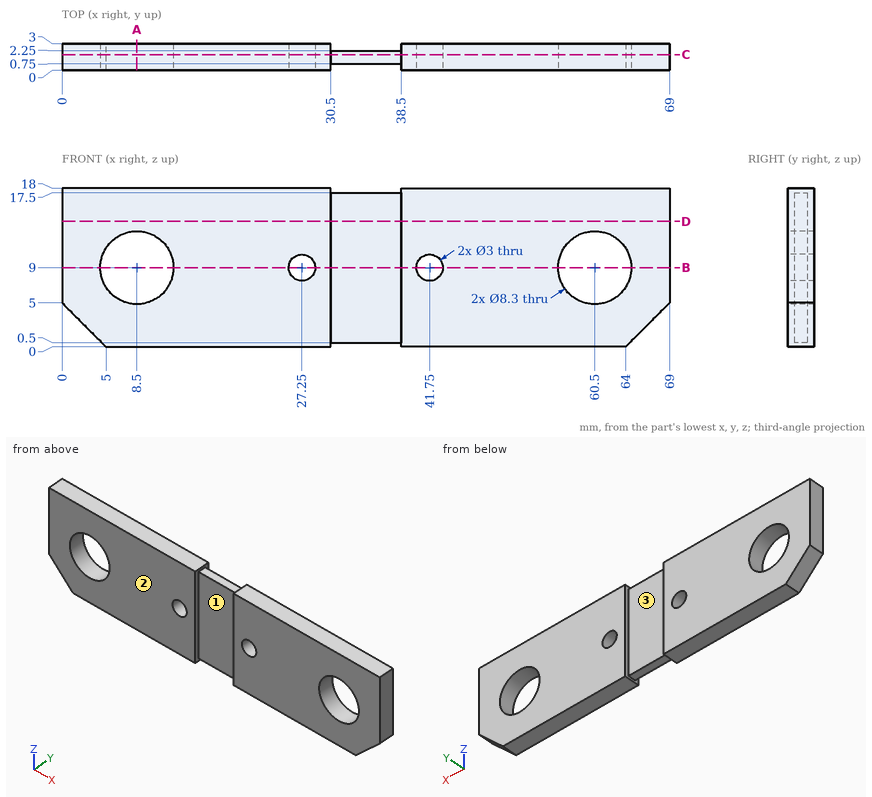
For this review, use the dimensioned drawing (mm, ordinates from the lowest corner) and the shaded views. Give positions to 0.01 mm unless a question says otherwise; leave off trailing zeros. Order: outer loops, then holes, each group sorted by start corner. A loop starts at its lowest first (then second) coordinate and runs counter-clockwise, first axis right, second up. Notation, with made-up numbers: M -23.5,5.5 L 14.5,5.5 A7 ccw 14.5,16.5 Z; hole C 89,86 d8. An arc over 180 degrees is marked long. One line per question, with ' | ' between items. Start each with the question number.
1) Consider section B-B, the plane z = 9. Give the boundary of the cut face in (x, y).
2) Consider section D-D, the plane z = 14.25. Give the boundary of the cut face in (x, y).
3) Wall thickness on L1, parallel to X at y = 2.35, z = 9; L2, parallel to X at y = 1.8, z = 9; L3, parallel to Z at x = 60.5, y = 0.85: over which ranges is each line inside the solid? List them lowest first. Write a range as from..to.
4) Mouldability with a two-part tool opening along X and no side actions: class the marked faces 1, 2 and 3 as pulls with the +X half, pulls with the -X half, needs draft (parallel to the pull), parting line crosses it, or undercut.
5) Consider section C-C, the plane y = 1.8. Give the boundary of the cut face in (x, z), then the cut area to 3 significant figures.
6) Clearance check with flat-ended pins moving along their axes: P1, Ø2.5, axis at x = 33.5, z = 7, coming from the -Y side; P2, Ø2.5, axis at x = 27.25, z = 9, coming from the -Y side; P3, Ø1.2, axis at x = 35, y = 1.5, coming from the -Z side; P4, Ø2.5, axis at x = 33, z = 12.5, coming from the +Y side. State where each tip first meets the part, or that it passes through.
7) Consider section A-A, the plane x = 8.5. Give the boundary of the cut face in (y, z).
Found:
1) outline: M 0,0 L 4.35,0 L 4.35,3 L 0,3 Z; M 12.65,0 L 25.75,0 L 25.75,3 L 12.65,3 Z; M 28.75,0 L 30.5,0 L 30.5,0.75 L 38.5,0.75 L 38.5,0 L 40.25,0 L 40.25,3 L 38.5,3 L 38.5,2.25 L 30.5,2.25 L 30.5,3 L 28.75,3 Z; M 43.25,0 L 56.35,0 L 56.35,3 L 43.25,3 Z; M 64.65,0 L 69,0 L 69,3 L 64.65,3 Z
2) outline: M 0,0 L 30.5,0 L 30.5,0.75 L 38.5,0.75 L 38.5,0 L 69,0 L 69,3 L 38.5,3 L 38.5,2.25 L 30.5,2.25 L 30.5,3 L 0,3 Z
3) L1: x = 0..4.35, 12.65..25.75, 28.75..30.5, 38.5..40.25, 43.25..56.35, 64.65..69 | L2: x = 0..4.35, 12.65..25.75, 28.75..40.25, 43.25..56.35, 64.65..69 | L3: z = 0..4.85, 13.15..18
4) face 1: undercut | face 2: needs draft | face 3: undercut
5) outline: M 0,5 L 5,0 L 30.5,0 L 30.5,0.5 L 38.5,0.5 L 38.5,0 L 64,0 L 69,5 L 69,18 L 38.5,18 L 38.5,17.5 L 30.5,17.5 L 30.5,18 L 0,18 Z; hole C 8.5,9 d8.3; hole C 27.25,9 d3; hole C 41.75,9 d3; hole C 60.5,9 d8.3 | area: 1,090 mm²
6) P1: stops at y = 0.75 | P2: passes through | P3: stops at z = 0.5 | P4: stops at y = 2.25
7) outline: M 0,0 L 3,0 L 3,4.85 L 0,4.85 Z; M 0,13.15 L 3,13.15 L 3,18 L 0,18 Z
